Could you check a few things on this model? Use its own coordinates, in mm. Coordinates: 2 decimals unless noted, no trailing zeros. Write each loop counter-clockwise with the first axis right and the second up, starting at its lowest first coordinate (ties: lowest second). Pieces come first, ordered by that corner, then holes.
Autodesk Inventor part; units mm, degrees
ref_plane "YZ Plane" through (0, 0, 0) normal (1, 0, 0) x (0, 1, 0)
ref_plane "XZ Plane" through (0, 0, 0) normal (0, 1, 0) x (-1, 0, 0)
ref_plane "XY Plane" through (0, 0, 0) normal (0, 0, 1) x (1, 0, 0)
sketch "Sketch1" plane through (0, 0, 0) normal (0, 0, 1) x (1, 0, 0)
  circle A0 centre (0, 0) radius 4
  line L0 (0, 0) -> (48, 0)
  circle A1 centre (48, 0) radius 4
  line L1 (0, 0) -> (0, 10)
  line L2 (0, 10) -> (60, 10)
  line L3 (60, 10) -> (60, -10)
  line L4 (60, -10) -> (-5, -10)
  line L5 (-5, -10) -> (-5, 10)
  line L6 (-5, 10) -> (0, 10)
  dimension "d0" = 8
  dimension "d1" = 48
  dimension "d2" = 8
  dimension "d3" = 10
  dimension "d4" = 60
  dimension "d5" = 20
  dimension "d6" = 65
extrude "Extrusion1" add sketch "Sketch1" along normal blind 8
properties part number "plaque 2"
Item 1: I want a section at C-C, the plane z = 7. List the corners of the cut face in (x, y) for me, then the cut area to 3 significant figures.
Item 2: If I drill on line 1 along Y through (x, z) = (0, 4.5); line 2 along X through (y, z) = (-2.25, 7.5); line 3 along Y through (x, z) = (49.5, 3.75), over which ranges is the centre line in solid material (lowest first)?
Item 3: I want a section at A-A, the plane x = 48. List the corners of the cut face in (y, z) for me, then the cut area to 3 significant figures.
Item 4: If we mould it in two halves opening along X, with no side actions, what happens to faces 1 (the flat face through (27, 0, 0)), 2 (the flat face through (-5, 0, 4)), 3 (the cylindrical face through (44, 0, 4))? For each: released by +X, released by -X, zero draft, split by the parting line, or undercut.
Item 5: I want a section at B-B, the plane y = 0. List the corners of the cut face in (x, z) for me, then the cut area to 3 significant figures.
Taken from the geometry:
1. outline: (-5, -10) - (60, -10) - (60, 10) - (-5, 10) - close; hole circle Ø8 at (0, 0); hole circle Ø8 at (48, 0)
1. area: 1,200 mm2
2. line 1: y = -10 to -4, 4 to 10
2. line 2: x = -5 to -3.31, 3.31 to 44.69, 51.31 to 60
2. line 3: y = -10 to -3.71, 3.71 to 10
3. outline: (-10, 0) - (-4, 0) - (-4, 8) - (-10, 8) - close; (4, 0) - (10, 0) - (10, 8) - (4, 8) - close
3. area: 96.0 mm2
4. face 1: zero draft
4. face 2: released by -X
4. face 3: undercut
5. outline: (-5, 0) - (-4, 0) - (-4, 8) - (-5, 8) - close; (4, 0) - (44, 0) - (44, 8) - (4, 8) - close; (52, 0) - (60, 0) - (60, 8) - (52, 8) - close
5. area: 392 mm2
